Source: three-view drawing plus pictorial views. Frame: mm from the lowest corner of the part. A direction names the side the tool comes from. Coordinates: 2 decimals unless noted, no trailing zeros. Write each loop counter-clockwise with the first axis right and the second up, starting at its lowest first coordinate (ties: lowest second). Pieces come first, ordered by that corner, then holes. Notation, with made-up numbers: (36, 35) - (61, 35) arc R37 cw to (61, 71) - close; hole circle Ø4 at (36, 10). An arc over 180 degrees is marked (long way). Answer as a JSON object with one key per item and string values. Group by question number.
Item 1: Line query: line 1 along Y through (x, z) = (2, 5.5) (1 decimal); line 2 along X through (y, z) = (21, 6.25); line 3 along Z through (x, y) = (8.5, 12.5) (1 decimal). Output: solid intervals per line, ascending. Write a range as from..to.
Item 2: Section D-D on z = 10. Return loops of the section in (x, y) (1 decimal), and give its area (3 significant figures).
Item 3: Section C-C on y = 34. Return loops of the section in (x, z).
Item 4: Set-up query: the marked faces 1, 2 and 3. Return all of +Z, -Z, +X, -X, +Y, -Y with unobstructed straight access to the full face (end or side cutting, diameter ignored); none if empty.
Item 5: Section A-A on x = 5.5. Return loops of the section in (y, z) (1 decimal), and give its area (3 significant figures).
Item 6: Section B-B on z = 5.5. Return loops of the section in (x, y) (1 decimal), and give its area (3 significant figures).
Item 7: First-contact query: pin 1 Ø1.5 at (x, y) = (3.5, 14.5) entering from -Z; pin 2 Ø1 at (x, z) = (6, 6.5) entering from -Y; pin 3 Ø1.5 at (y, z) = (40, 4) entering from +X; pin 4 Ø1.5 at (x, y) = (2, 28.5) entering from -Z. Flat tips, straight axial feed; report the tip coordinate or a pass-through.
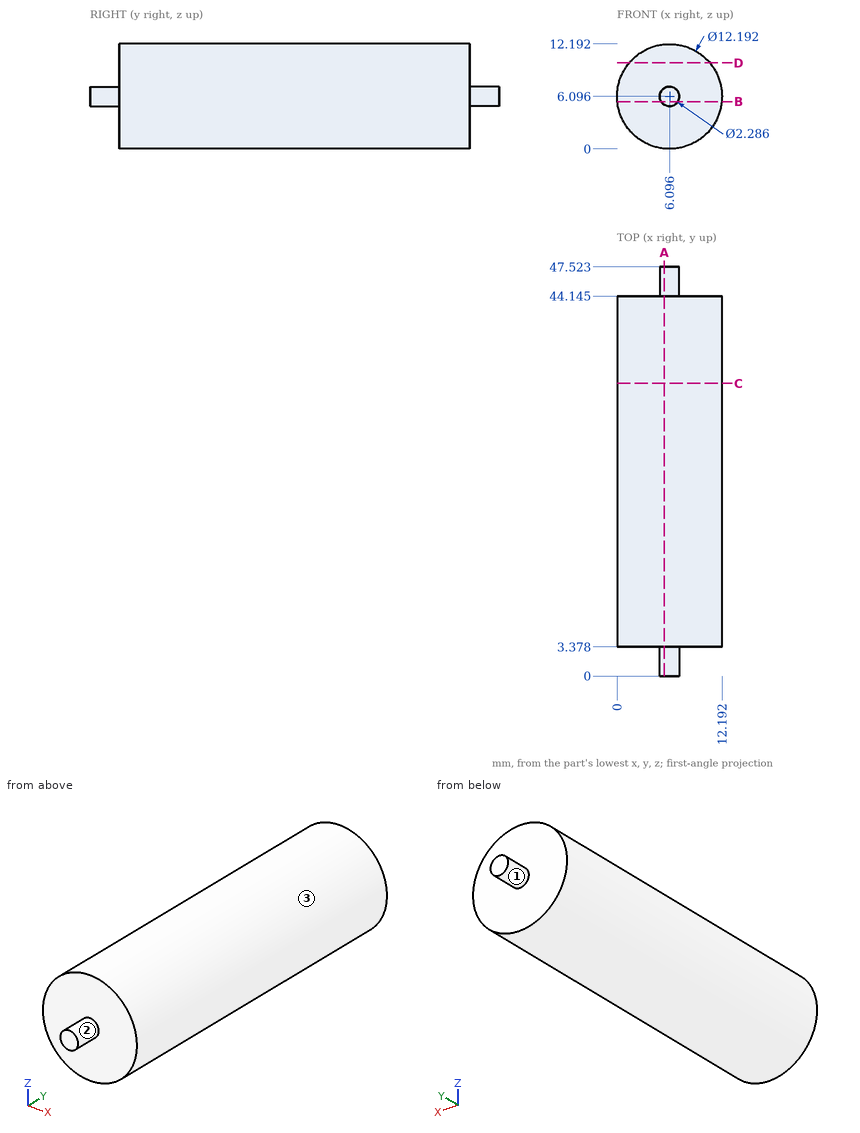
Checks:
{
 "1": {"line 1": "3.4..44.1", "line 2": "0..12.19", "line 3": "0.5..11.7"},
 "2": {"outline": "(1.4, 3.4) - (10.8, 3.4) - (10.8, 44.1) - (1.4, 44.1) - close", "area": "382 mm^2"},
 "3": {"outline": "circle Ø12.19 at (6.1, 6.1)"},
 "4": {"face 1": "+Y", "face 2": "-Y", "face 3": "+Y, -Y"},
 "5": {"outline": "(0, 5.1) - (3.4, 5.1) - (3.4, 0) - (44.1, 0) - (44.1, 5.1) - (47.5, 5.1) - (47.5, 7.1) - (44.1, 7.1) - (44.1, 12.2) - (3.4, 12.2) - (3.4, 7.1) - (0, 7.1) - close", "area": "508 mm^2"},
 "6": {"outline": "(0, 3.4) - (5.1, 3.4) - (5.1, 0) - (7.1, 0) - (7.1, 3.4) - (12.2, 3.4) - (12.2, 44.1) - (7.1, 44.1) - (7.1, 47.5) - (5.1, 47.5) - (5.1, 44.1) - (0, 44.1) - close", "area": "508 mm^2"},
 "7": {"pin 1": "z = 0.29", "pin 2": "y = 0", "pin 3": "x = 12.04", "pin 4": "z = 1"}
}
